Work out the finished part from the listing and answer in its coordinate system (mm). A direction names the side the tool comes from. Give positions to 0.01 mm unless a question says otherwise; leave off trailing zeros. Write each loop counter-clockwise with the first axis right and the second up, starting at its lowest first coordinate (ties: lowest second). Pieces come first, ordered by that corner, then holes. Notation, with made-up numbers: (84, 27.25) -> (123, 27.25) arc R23 cw to (123, 65.25) -> close; hole circle Ø6 at (37, 82). An arc over 180 degrees is marked (long way). Use a Markdown table: item, result. Add a question column.
Q1. For a pull along Y with two mould halves and no side action, classify faces 1 (the face through (-74.39, 17.14, 9.04)), 2 (the face through (-76.2, 0, 9)), 3 (the face through (-57.15, 3, 9)) as pulls with the +Y half, pulls with the -Y half, needs draft (parallel to the pull), parting line crosses it, or undercut.
Q2. Section A-A, the plane x = 4 is taken. Give the vertices of the cut face in (y, z) (3 decimals), plus the area to 3 significant figures.
Q3. This flat-tipped pin is pushed along its axis until it touches: pin 1 Ø3 at (y, z) = (15, 16) entering from -X. Where does it stop, or does it pass through?
Q4. Section C-C, the plane z = 5 is taken. Give the vertices of the cut face in (x, y) (3 decimals).
Q5. For faces 4 (the face through (-55.24, -7.714, 8.791)), 5 (the face through (-1, -12, 0)), determine the directions among +Z, -Z, +X, -X, +Y, -Y from which every point of the face is accessible in a straight line to the end or side of a thin tool.
Q6. Consider line 1 (Y direction, x = -46.5, z = 8.5) (3 decimals); line 2 (X direction, y = -2.5, z = 16.75); line 3 (X direction, y = 8.5, z = 2.75). Determine where each line is inside the solid, lowest interval first.
Q7. Section B-B, the plane y = 1 is taken. Give the vertices of the cut face in (x, z).
from build123d import *

# Parameters (mm, degrees)
SKETCH1_W           = 152.4
SKETCH1_H           = 38.1
BOSS_EXTRUDE1_DEPTH = 17.8308
SKETCH2_W           = 114.3
SKETCH2_H           = 25.4
CUT_EXTRUDE1_DEPTH  = 81.543652317
FILLET1_R           = 6.35
SKETCH3_R           = 3.175
CUT_EXTRUDE2_DEPTH  = 81.543652317


with BuildPart() as part:
    # Sketch1 → Boss-Extrude1 (new body)
    with BuildSketch(Plane.XY):
        Rectangle(SKETCH1_W, SKETCH1_H)
    extrude(amount=BOSS_EXTRUDE1_DEPTH)

    # Sketch2 → Cut-Extrude1 (cut, through all)
    with BuildSketch(Plane.XY.offset(17.8308)):
        with Locations((0, 3.175)):
            Rectangle(SKETCH2_W, SKETCH2_H)
    extrude(amount=-CUT_EXTRUDE1_DEPTH, mode=Mode.SUBTRACT)

    # Fillet1
    fillet1_edges = [part.edges().sort_by_distance(p)[0] for p in [
        (-57.15, -9.525, 8.9154),
        (-57.15, 15.875, 8.9154),
        (57.15, 15.875, 8.9154),
        (57.15, -9.525, 8.9154),
        (-76.2, 19.05, 8.9154),
        (76.2, 19.05, 8.9154),
        (76.2, -19.05, 8.9154),
        (-76.2, -19.05, 8.9154),
    ]]
    fillet(fillet1_edges, radius=FILLET1_R)

    # Sketch3 → Cut-Extrude2 (cut, through all)
    with BuildSketch(Plane.XY.offset(17.8308)):
        with Locations((-66.675, 6.71302)):
            Circle(SKETCH3_R)
        with Locations((66.675, 6.71302)):
            Circle(SKETCH3_R)
    extrude(amount=-CUT_EXTRUDE2_DEPTH, mode=Mode.SUBTRACT)


solid = part.part
Result set:
| question | item | result |
|---|---|---|
| 1 | face 1 | pulls with the +Y half |
| 1 | face 2 | needs draft |
| 1 | face 3 | undercut |
| 2 | outline | (-19.05, 0) -> (-9.525, 0) -> (-9.525, 17.831) -> (-19.05, 17.831) -> close; (15.875, 0) -> (19.05, 0) -> (19.05, 17.831) -> (15.875, 17.831) -> close |
| 2 | area | 226 mm2 |
| 3 | pin 1 | stops at x = -76.15 |
| 4 | outline | (-76.2, -12.7) arc R6.35 ccw to (-69.85, -19.05) -> (69.85, -19.05) arc R6.35 ccw to (76.2, -12.7) -> (76.2, 12.7) arc R6.35 ccw to (69.85, 19.05) -> (-69.85, 19.05) arc R6.35 ccw to (-76.2, 12.7) -> close; hole circle Ø6.35 at (-66.675, 6.713); hole (-57.15, -3.175) arc R6.35 ccw to (-50.8, -9.525) -> (50.8, -9.525) arc R6.35 ccw to (57.15, -3.175) -> (57.15, 9.525) arc R6.35 ccw to (50.8, 15.875) -> (-50.8, 15.875) arc R6.35 ccw to (-57.15, 9.525) -> close; hole circle Ø6.35 at (66.675, 6.713) |
| 5 | face 4 | +Z, -Z |
| 5 | face 5 | -Z, +X, -X, +Y, -Y |
| 6 | line 1 | y = -19.05 to -9.525, 15.875 to 19.05 |
| 6 | line 2 | x = -76.2 to -57.15, 57.15 to 76.2 |
| 6 | line 3 | x = -76.2 to -69.3, -64.05 to -57.15, 57.15 to 64.05, 69.3 to 76.2 |
| 7 | outline | (-76.2, 0) -> (-57.15, 0) -> (-57.15, 17.83) -> (-76.2, 17.83) -> close; (57.15, 0) -> (76.2, 0) -> (76.2, 17.83) -> (57.15, 17.83) -> close |
